from build123d import *

# Parameters (mm, degrees)
SKETCH1_W                 = 155
SKETCH1_H                 = 45
BOSS_EXTRUDE1_DEPTH       = 10
SKETCH2_W                 = 65
SKETCH2_H                 = 45
BOSS_EXTRUDE2_DEPTH       = 12
CUT_EXTRUDE1_DEPTH        = 59
SKETCH4_W                 = 55
SKETCH4_H                 = 30
CUT_EXTRUDE2_DEPTH        = 12
M5_TAPPED_HOLE1_D         = 4.2
M3_TAPPED_HOLE1_D         = 2.5
M3_TAPPED_HOLE1_DEPTH     = 7.5
M3_TAPPED_HOLE1_TIP       = 0.751075774
HOLE_WIZARD_M4_1_D        = 3.3
CHAMFER1_SIZE             = 5
FILLET_1_R                = 5
FILLET_2_R                = 2
HOLE_WIZARD_1_D           = 8.4
HOLE_WIZARD_1_CBORE_D     = 15
HOLE_WIZARD_1_CBORE_DEPTH = 7


with BuildPart() as part:
    # Sketch1 → Boss-Extrude1 (new body)
    with BuildSketch(Plane.XY):
        with Locations((31.848694107, 0)):
            Rectangle(SKETCH1_W, SKETCH1_H)
    extrude(amount=BOSS_EXTRUDE1_DEPTH)

    # Sketch2 → Boss-Extrude2 (add)
    with BuildSketch(Plane.XY.offset(10)):
        with Locations((76.848694107, 0)):
            Rectangle(SKETCH2_W, SKETCH2_H)
    extrude(amount=BOSS_EXTRUDE2_DEPTH)

    # Sketch3 → Cut-Extrude1 (cut)
    with BuildSketch(Plane.XY.offset(22)):
        with BuildLine():
            Line((64.348694107, 10), (89.348694107, 10))
            ThreePointArc((89.348694107, 10), (99.348694107, 0), (89.348694107, -10))
            Line((89.348694107, -10), (64.348694107, -10))
            ThreePointArc((64.348694107, -10), (54.348694107, 0), (64.348694107, 10))
        make_face()
    extrude(amount=-CUT_EXTRUDE1_DEPTH, mode=Mode.SUBTRACT)

    # Sketch4 → Cut-Extrude2 (cut)
    with BuildSketch(Plane.XY.offset(22)):
        with Locations((76.848694107, 0)):
            Rectangle(SKETCH4_W, SKETCH4_H)
    extrude(amount=-CUT_EXTRUDE2_DEPTH, mode=Mode.SUBTRACT)

    # M5 Tapped Hole1 (through all)
    with Locations(Plane.ZY.offset(-44.348694107)):
        with Locations((16, 0)):
            Hole(M5_TAPPED_HOLE1_D / 2)

    # M3 Tapped Hole1
    with Locations(Plane.XY.offset(22)):
        with Locations((104.348694107, -17.5), (104.348694107, 17.5), (49.348694107, -17.5), (49.348694107, 17.5)):
            Hole(M3_TAPPED_HOLE1_D / 2, depth=M3_TAPPED_HOLE1_DEPTH)
            with Locations((0, 0, -(M3_TAPPED_HOLE1_DEPTH + M3_TAPPED_HOLE1_TIP / 2))):  # 118° drill point
                Cone(0, M3_TAPPED_HOLE1_D / 2, M3_TAPPED_HOLE1_TIP, mode=Mode.SUBTRACT)

    # M4 螺纹孔1 (through all)
    with Locations(Plane(origin=(0, -22.5, 0), x_dir=(-1, 0, 0), z_dir=(0, -1, 0))):
        with Locations((-94.348694107, -15), (-54.348694107, -15)):
            Hole(HOLE_WIZARD_M4_1_D / 2)

    # Chamfer1
    chamfer1_edges = [part.edges().sort_by_distance(p)[0] for p in [
        (-45.651305893, -22.5, 5),
        (-45.651305893, 22.5, 5),
    ]]
    chamfer(chamfer1_edges, length=CHAMFER1_SIZE)

    # 圆角1
    fillet_1_edges = [part.edges().sort_by_distance(p)[0] for p in [
        (109.348694107, 22.5, 11),
        (109.348694107, -22.5, 11),
    ]]
    fillet(fillet_1_edges, radius=FILLET_1_R)

    # 圆角2
    fillet_2_edges = [part.edges().sort_by_distance(p)[0] for p in [
        (49.348694107, -15, 16),
        (49.348694107, 15, 16),
        (104.348694107, 15, 16),
        (104.348694107, -15, 16),
    ]]
    fillet(fillet_2_edges, radius=FILLET_2_R)

    # 打孔尺寸(%根据)内六角圆柱头螺钉的类型1 (through all)
    with Locations(Plane.XY.offset(10)):
        with Locations((21.848694107, 0), (-23.151305893, 0)):
            CounterBoreHole(HOLE_WIZARD_1_D / 2, HOLE_WIZARD_1_CBORE_D / 2, HOLE_WIZARD_1_CBORE_DEPTH)


solid = part.part
Can you work these out from the model? Positions are in its coordinate system, mm. A direction names the side the tool comes from. Coordinates: 2 decimals unless noted, no trailing zeros. Write each loop counter-clockwise with the first axis right and the second up, starting at its lowest first coordinate (ties: lowest second). Pieces come first, ordered by that corner, then holes. Notation, with made-up numbers: (79, -14) -> (114, -14) arc R11 cw to (114, -9) -> close; hole circle Ø5 at (49, 8.5). An arc over 180 degrees is marked (long way). Write each question's results on one line, items separated by ' | '. Start each with the question number.
Q1. On a 3-axis mill with a long thin cutter (end or side, diameter ignored), from which of +Z, -Z, +X, -X, +Y, -Y can I reach the whole of each face in a straight line? I mean faces 1 (the face through (76, 15, 16)), 2 (the face through (77, 10, 5)), 3 (the face through (-1, 0, 10)). Say none if no direction works.
Q2. I'm going to push flat-ended pins straight in: pin 1 (12 mm diameter, centred on x = -23.15, y = 0, fed in from +Z); pin 2 (2.5 mm diameter, centred on x = 94.35, z = 15, fed in from +Y); pin 3 (22.5 mm diameter, centred on x = 4.5, y = 7.5, fed in from +Z); pin 4 (3 mm diameter, centred on y = -10.5, z = 15, fed in from -X). Where does each tip first touch, or does it pass through?
Q3. Imagine slicing it at B-B (y = 0). State how many separate pieces and enclosed holes the cut face has, then the cut area to 3 significant figures.
Q4. Imagine slicing it at C-C (x = 34). Write out the boundary of the cut face in (y, z), then the cut area to 3 significant figures.
Q5. We'd pull the mould along Z, two halves only. Please class faces 4 (the face through (46.88, 0.09, 18.1)), 5 (the face through (14.356, 0.33, 6.549)), 6 (the face through (96, -19, 15)), 7 (the face through (-20, -3, 3)): +Z half, -Z half, draft (parallel to the pull), parting line (faces both ways), or undercut.
Q6. Imagine slicing it at A-A (x = 84). Write out the boundary of the cut face in (y, z), then the cut area to 3 significant figures.
Q7. If I drill on probe 1 along X at (y, z) = (17.5, 18); probe 2 along X at (y, z) = (-3.5, 2.25); probe 3 along X at (y, z) = (3.5, 15.5), over which ranges is the centre line in solid material (lowest first)?
Taken from the geometry:
1) face 1: +Z | face 2: +Z, -Z | face 3: +Z, -X, +Y, -Y
2) pin 1: stops at z = 3 | pin 2: passes through | pin 3: stops at z = 10 | pin 4: stops at x = 44.35
3) separate pieces: 6 | enclosed holes: 0 | area: 918 mm^2
4) outline: (-22.5, 0) -> (22.5, 0) -> (22.5, 10) -> (-22.5, 10) -> close | area: 450 mm^2
5) face 4: undercut | face 5: draft | face 6: undercut | face 7: +Z half
6) outline: (-22.5, 0) -> (-10, 0) -> (-10, 10) -> (-15, 10) -> (-15, 22) -> (-22.5, 22) -> close; (10, 0) -> (22.5, 0) -> (22.5, 22) -> (15, 22) -> (15, 10) -> (10, 10) -> close | area: 430 mm^2
7) probe 1: x = 44.35 to 48.1, 50.6 to 103.1, 105.6 to 109.35 | probe 2: x = -45.65 to -25.47, -20.83 to 19.53, 24.17 to 54.98, 98.72 to 109.35 | probe 3: x = 44.35 to 49.35, 104.35 to 109.35
